Part model, mm, in its own coordinate system. A direction names the side the tool comes from. Round coordinates to 2 decimals unless told otherwise and drop trailing zeros. Loops run counter-clockwise (first coordinate to the right, second up) from the corner with the lowest first, then second, coordinate; pieces in that order, holes last. Notation, with made-up numbers: M 55.5,54.5 L 104.5,54.5 A33 ccw 104.5,87.5 Z; hole C 62,74.5 d1. An arc over 180 degrees is marked long. Answer as CSV lines item,"result". Start each with the question number.
Item 1: Band-saw the part on A-A (x = 0). Give the cut face in (y, z), and give its area (3 significant figures).
Item 2: Which spindle directions (+Z, -Z, +X, -X, +Y, -Y) get a long thin tool onto all of the face, cutting with end or side? Do faces 4 (the flat face through (-8, 4, 2)), 5 (the flat face through (8, -9, 1)). Say none if no direction does.
Item 3: Drop flat-ended pins along their axis: pin 1 Ø1 at (y, z) = (-7.5, 0.5) entering from +X; pin 2 Ø6 at (x, y) = (8, -1) entering from +Z; pin 3 Ø1 at (y, z) = (-3.5, 0.5) entering from -X; pin 4 Ø1 at (x, y) = (11, 8) entering from +Z. Give the stop position or say it passes through.
Item 4: Mould opens along Y. For faces 1 (the cylindrical face through (-6.944, 5.324, 0.986)), 2 (the flat face through (6.5, -6.5, 0)), 3 (the cylindrical face through (-14.985, -0.66, 0.493)) say: pulls with the +Y half, pulls with the -Y half, needs draft (parallel to the pull), parting line crosses it, or undercut.
Item 5: Wall check: line 1 (Y direction, x = 0, z = 0.4); line 2 (Z direction, x = -10, y = -10); line 3 (X direction, y = -4.25, z = 1.9). Give the ranges that are in metal, low to high.
Item 6: Band-saw the part on C-C (x = 12.75). Give the cut face in (y, z), and give its area (3 significant figures).
Autodesk Inventor part; units mm, degrees
ref_plane "YZ Plane" through (0, 0, 0) normal (1, 0, 0) x (0, 1, 0)
ref_plane "XZ Plane" through (0, 0, 0) normal (0, 1, 0) x (-1, 0, 0)
ref_plane "XY Plane" through (0, 0, 0) normal (0, 0, 1) x (1, 0, 0)
sketch "Sketch1" plane through (0, 0, 0) normal (0, 0, 1) x (1, 0, 0)
  circle A0 centre (0, 0) radius 8.75
  circle A1 centre (0, 0) radius 15
  circle A2 centre (0, 0) radius 9.75
  dimension "d0" = 17.5
  dimension "d1" = 30
  dimension "d2" = 1
extrude "Extrusion1" add sketch "Sketch1" along normal blind 1 contours A1
extrude "Extrusion2" add sketch "Sketch1" along normal blind 2 contours A2
fillet "Fillet1" radius 2 1 edges at (-9.75, 0, 1)
properties part number "Retenedor"
Answer block:
1,outline,"M -15,0 L -8.75,0 L -8.75,2 L -9.75,2 A2 cw -11.48,1 L -15,1 Z; M 8.75,0 L 15,0 L 15,1 L 11.48,1 A2 cw 9.75,2 L 8.75,2 Z"
1,area,"15.5 mm^2"
2,face 4,"+Z, +X, -X, +Y, -Y"
2,face 5,"+Z"
3,pin 1,"stops at x = 13.27"
3,pin 2,"stops at z = 2"
3,pin 3,"stops at x = -14.7"
3,pin 4,"stops at z = 1"
4,face 1,"undercut"
4,face 2,"needs draft"
4,face 3,"parting line crosses it"
5,line 1,"y = -15 to -8.75, 8.75 to 15"
5,line 2,"z = 0 to 1"
5,line 3,"x = -8.84 to -7.65, 7.65 to 8.84"
6,outline,"M -7.9,0 L 7.9,0 L 7.9,1 L -7.9,1 Z"
6,area,"15.8 mm^2"
